Autodesk Inventor part; units mm, degrees
ref_plane "Arbeitsebene1" through (0, 0, 1.5) normal (0, 0, 1) x (1, 0, 0)
ref_plane "Arbeitsebene2" through (0, -1.5, 0) normal (0, 1, 0) x (-1, 0, 0)
ref_plane "YZ Plane" through (0, 0, 0) normal (1, 0, 0) x (0, 1, 0)
sketch "Skizze" plane through (0, 0, 0) normal (1, 0, 0) x (0, 1, 0)
  circle A0 centre (0, 0) radius 1.5
  dimension "d1" = 3
extrude "Körper" add sketch "Skizze" along normal blind 16
chamfer "Fase1" distance 0.5 angle 15 1 edges at (0, -1.5, 0) measured on face at (10.6667, 1.4951, -0.1207)
chamfer "Skizze2" distance 0.5 angle 15 1 edges at (16, -1.5, 0) measured on face at (10.8333, 1.4951, -0.1207)
ref_plane "Arbeitsebene1" through (0, 0, 1.5) normal (0, 0, 1) x (1, 0, 0)
sketch "Skizze3" plane through (0, 0, 1.5) normal (0, 0, 1) x (1, 0, 0)
  line L0 (0, -1.366) -> (0, 1.366)
  point P0 (0, 0)
  point P1 (5.5, 0)
  point P2 (0, 0)
  dimension "d18" = 5.5
hole "Bohrung1" at (5.5, 0, 1.5) direction (0, 0, -1) diameter 0.5 end through all
sketch "Skizze4" plane through (0, 0, 0) normal (0, 1, 0) x (-1, 0, 0)
  line L0 (-0.5, 1.5) -> (-15.5, 1.5)
  line L1 (-4.5, 1.5) -> (-4.5, 0.5)
  line L2 (-4.5, 0.5) -> (-6.5, 0.5)
  line L3 (-6.5, 0.5) -> (-6.5, 1.5)
  line L4 (0, 1.366) -> (0, -1.366)
  line L5 (-0.5, -1.5) -> (-15.5, -1.5)
  point P0 (0, 0)
  point P1 (-5.5, 0.5)
  dimension "d26" = 2
  dimension "d27" = 5.5
  dimension "d28" = 1
extrude "Extrusion2" cut sketch "Skizze4" along normal through all both and the other way through all
ref_plane "Arbeitsebene2" through (0, -1.5, 0) normal (0, 1, 0) x (-1, 0, 0)
sketch "Skizze5" plane through (0, -1.5, 0) normal (0, 1, 0) x (-1, 0, 0)
  line L0 (-16, -1.366) -> (-16, 1.366)
  line L1 (-13, 2.5) -> (-16, 2.5)
  line L2 (-16, 2.5) -> (-16, -2.5)
  line L3 (-16, -2.5) -> (-13, -2.5)
  line L4 (-13, -2.5) -> (-13, 2.5)
  point P0 (0, 0)
  point P1 (-16, 0)
  dimension "d32" = 3
  dimension "d33" = 5
extrude "Extrusion3" cut sketch "Skizze5" along normal blind 0.5
sketch "Skizze6" plane through (0, 0, 0) normal (0, 1, 0) x (-1, 0, 0)
  line L0 (-0.5, 1.5) -> (-15.5, 1.5)
  line L1 (-1, 1.5) -> (-1, 0.75)
  line L2 (-1, 0.75) -> (-2, 0.75)
  line L3 (-2, 0.75) -> (-2, 1.5)
  line L4 (0, 0) -> (-4.4819, 0)
  dimension "d36" = 1
  dimension "d37" = 1
  dimension "d38" = 0.75
revolve "Umdrehung1" cut sketch "Skizze6" angle 360 about axis through (0, 0, 0) along (1, 0, 0)
equation "\"d1\" = NND"
equation "\"d8\" = PHH"
equation "\"d9\" = FAWI"
equation "\"d12\" = PHH"
equation "\"d4\" = PHH"
equation "\"d5\" = FAWI"
equation "\"d11\" = PHH"
equation "\"NND\" = 3"
equation "\"NLG\" = 8"
equation "\"PHH\" = 0.5"
equation "\"FAWI\" = 15deg"
equation "\"KAH\" = 0"
properties part number "ISO 2338 - 3 m6 x 8" material "Edelstahl, austenitisch"
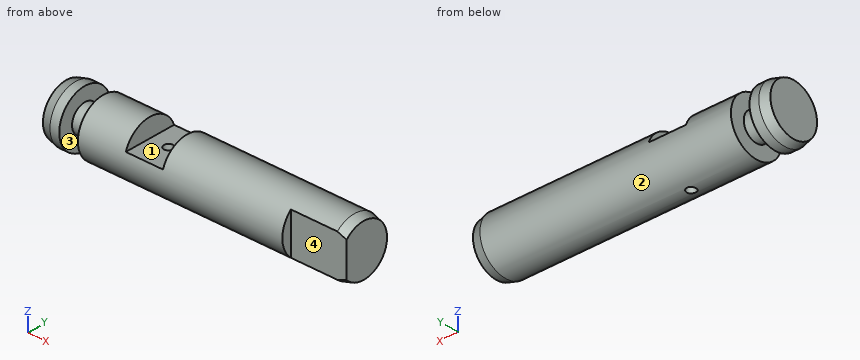
Geometry check sheet. Reference: the model listing, model coordinates, mm. Face numbers are marked on the shaded views. A direction names the side the tool comes from. Give positions to 0.01 mm unless a question says otherwise; leave off trailing zeros. Order: outer loops, then holes, each group sorted by start corner. A loop starts at its lowest first (then second) coordinate and runs counter-clockwise, first axis right, second up.
1. Sectioned sample at D-D (x = 14). Record the boundary of the cut face in (y, z).
Completed:
outline: (-1, -1.12) arc R1.5 ccw (long way) to (-1, 1.12) - close
2. Sectioned sample at A-A (z = 0). Record the boundary of the cut face in (x, y), then the cut area to 3 significant figures.
Completed:
outline: (0, -1.37) - (0.5, -1.5) - (1, -1.5) - (1, -0.75) - (2, -0.75) - (2, -1.5) - (13, -1.5) - (13, -1) - (16, -1) - (16, 1.37) - (15.5, 1.5) - (2, 1.5) - (2, 0.75) - (1, 0.75) - (1, 1.5) - (0.5, 1.5) - (0, 1.37) - close; hole circle Ø0.5 at (5.5, 0)
area: 44.7 mm2
3. Sectioned sample at B-B (y = 0). Record the boundary of the cut face in (x, z), then the cut area to 3 significant figures.
Completed:
outline: (0, -1.37) - (0.5, -1.5) - (1, -1.5) - (1, -0.75) - (2, -0.75) - (2, -1.5) - (5.25, -1.5) - (5.25, 0.5) - (4.5, 0.5) - (4.5, 1.5) - (2, 1.5) - (2, 0.75) - (1, 0.75) - (1, 1.5) - (0.5, 1.5) - (0, 1.37) - close; (5.75, -1.5) - (15.5, -1.5) - (16, -1.37) - (16, 1.37) - (15.5, 1.5) - (6.5, 1.5) - (6.5, 0.5) - (5.75, 0.5) - close
area: 43.4 mm2
4. Access from +Z, -Z, +X, -X, +Y, -Y to the whole of each face (thin tool, end or side, straight path). Record for the marked faces 1, 2, 3 and 4.
Completed:
face 1: +Z, +Y, -Y
face 2: +X, -X
face 3: none
face 4: +Z, -Z, +X, -Y
5. Sectioned sample at C-C (x = 5.5). Record the boundary of the cut face in (y, z), then the cut area to 3 significant figures.
Completed:
outline: (-1.41, 0.5) arc R1.5 ccw to (-0.25, -1.48) - (-0.25, 0.5) - close; (0.25, -1.48) arc R1.5 ccw to (1.41, 0.5) - (0.25, 0.5) - close
area: 4.01 mm2
6. Depth check by flat-ended pin: pin 1 (1 mm diameter, centred on x = 5.5, y = 0, fed in from +Z); pin 2 (0.6 mm diameter, centred on y = -1.5, z = 0, fed in from +X). Enter the tip coordinate at first touch or a pass-through.
Completed:
pin 1: stops at z = 0.5
pin 2: stops at x = 13
7. Scan lines: line 1 (X direction, y = 0.5, z = 0.65); line 2 (X direction, y = 0, z = 0); line 3 (Z direction, x = 3.75, y = 1.3). Record each from-to range of solid material in increasing order.
Completed:
line 1: x = 0 to 1, 2 to 4.5, 6.5 to 16
line 2: x = 0 to 5.25, 5.75 to 16
line 3: z = -0.75 to 0.75
